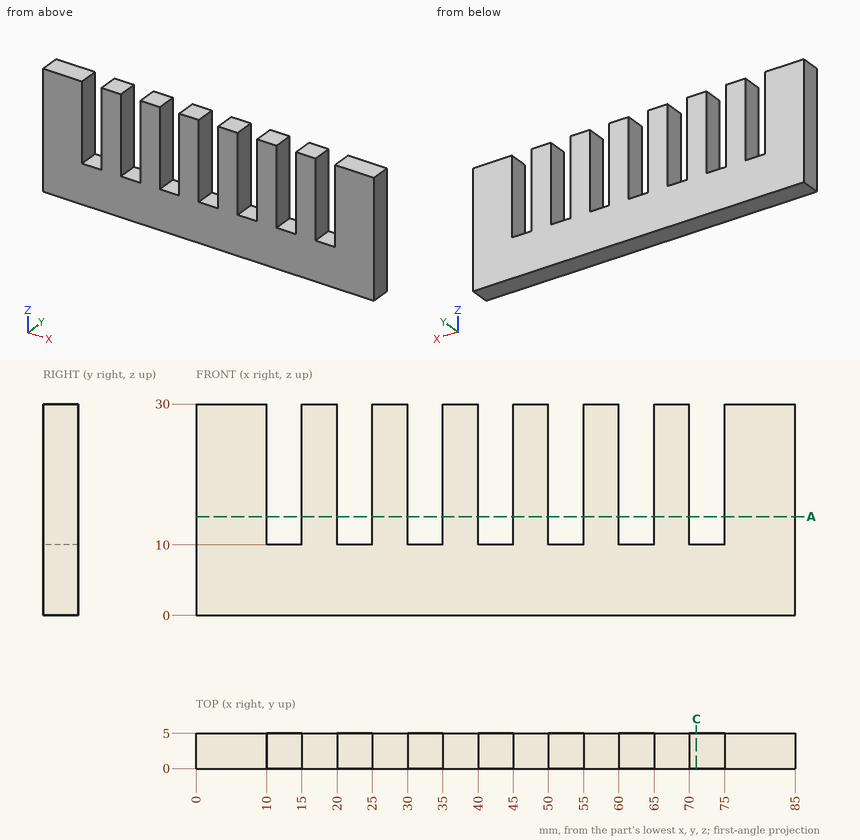
Check sheet for the drawn part. Datum: minimum x, y, z corner. Units: mm. Give positions to 0.01 mm unless a question says otherwise; leave off trailing zeros. Order: outer loops, then holes, each group sorted by start corner. A loop starts at its lowest first (then second) coordinate and runs counter-clockwise, first axis right, second up. Notation, with made-up numbers: (-27, 0) -> (-22, 0) arc R22 ccw to (-22, 16) -> close; hole circle Ø10 at (-32, -14.75). An arc over 180 degrees is marked (long way). Return JSON: item names as keys, results as strings.
1. Material ranges on probe 1 along Z at (x, y) = (13.5, 1.4), recorded low to high. Write a range as [from, to].
From the geometry:
{"probe 1": "[0, 10]"}
2. Go/stop test with a flat-tipped pin: P1, Ø2.5, axis at x = 62.5, y = 1.5, coming from the +Z side. Record where the tip stops, or that it passes through.
From the geometry:
{"P1": "z = 10"}
3. Cross-section at A-A, the plane z = 14. Count the separate pieces of the cut face and the enclosed holes in it, plus the area to 3 significant figures.
From the geometry:
{"separate pieces": "8", "enclosed holes": "0", "area": "250 mm^2"}
4. Cross-section at C-C, the plane x = 71. Record the cut outline in (y, z).
From the geometry:
{"outline": "(0, 0) -> (5, 0) -> (5, 10) -> (0, 10) -> close"}
